from build123d import *

# Parameters (mm, degrees)
SKETCH_15_W          = 13
SKETCH_15_H          = 25
EXTRUDE_4_DEPTH      = 20
CUT_EXTRUDE_START    = 1
SKETCH_16_W          = 12
SKETCH_16_H          = 23
CUT_EXTRUDE_47_DEPTH = 24.6018292
CUT_EXTRUDE_48_DEPTH = 25.6018292


with BuildPart() as part:
    # 스케치15 → 보스-돌출4 (new body)
    with BuildSketch(Plane(origin=(0, 0, 0), x_dir=(1, 0, 0), z_dir=(0, 1, 0))):
        with Locations((0.5, 0)):
            Rectangle(SKETCH_15_W, SKETCH_15_H)
    extrude(amount=EXTRUDE_4_DEPTH)

    # 스케치16 → 컷-돌출47 (cut, through all)
    with BuildSketch(Plane(origin=(0, 0, 0), x_dir=(1, 0, 0), z_dir=(0, 1, 0)).offset(CUT_EXTRUDE_START)):
        with Locations((1, 0)):
            Rectangle(SKETCH_16_W, SKETCH_16_H)
    extrude(amount=CUT_EXTRUDE_47_DEPTH, mode=Mode.SUBTRACT)

    # 스케치17 → 컷-돌출48 (cut, through all)
    with BuildSketch(Plane(origin=(0, 0, 0), x_dir=(1, 0, 0), z_dir=(0, 1, 0))):
        with BuildLine():
            Line((-5, 2.5), (7, 2.5))
            Line((7, 2.5), (7, -5.5))
            ThreePointArc((7, -5.5), (1, -11.5), (-5, -5.5))
            Line((-5, -5.5), (-5, 2.5))
        make_face()
    extrude(amount=CUT_EXTRUDE_48_DEPTH, mode=Mode.SUBTRACT)


solid = part.part
Model file for the job. Use its own axes, mm. A direction names the side the tool comes from. Give positions to 0.01 mm unless a question says otherwise; leave off trailing zeros. Loops run counter-clockwise (first coordinate to the right, second up) from the corner with the lowest first, then second, coordinate; pieces in that order, holes last. Notation, with made-up numbers: (-29, -20.75) -> (-9, -20.75) arc R30 ccw to (-9, 15.25) -> close; hole circle Ø9 at (15.25, 48.5). An arc over 180 degrees is marked (long way). Use a Markdown table: item, result. Add a question column.
(1) Slice it at B-B on z = 10.75. List the corners of the cut face in (x, y).
(2) Slice it at D-D on z = -8. List the corners of the cut face in (x, y).
(3) Drop a flat-ended pin along its axis: pin 1 Ø4.5 at (x, z) = (3.5, -8.5) entering from +Y. Give the stop position or say it passes through.
(4) Slice it at C-C on y = 13.5. List the corners of the cut face in (x, z), and give its area (3 significant figures).
(5) Slice it at A-A on x = -4.25. List the corners of the cut face in (y, z), and give its area (3 significant figures).
(6) Wall check: line 1 along Z through (x, y) = (5.75, 15.25); line 2 along X through (y, z) = (7, 7); line 3 along Y through (x, z) = (-4.75, -7.5). Give the ranges that are in metal, low to high.
(7) Tool access for faces 1 (the flat face through (0.9, 0.5, -2.5)), 2 (the flat face through (0, 10, 12.5)), 3 (the flat face through (6, 1, 10)): list every direction of +Z, -Z, +X, -X, +Y, -Y with a clear straight run to the whole face (end or side of a thin tool).
(8) Mould opens along X. For faces 4 (the cylindrical face through (1.1, 0.5, 11.5)), 5 (the flat face through (7, 8, 12)), 6 (the flat face through (0, 0, -3)) say: +X half, -X half, draft (parallel to the pull), parting line (faces both ways), or undercut.
Filled sheet:
| question | item | result |
|---|---|---|
| 1 | outline | (-6, 0) -> (-1.9, 0) -> (-1.9, 1) -> (-5, 1) -> (-5, 20) -> (-6, 20) -> close; (3.9, 0) -> (7, 0) -> (7, 1) -> (3.9, 1) -> close |
| 2 | outline | (-6, 0) -> (7, 0) -> (7, 1) -> (-5, 1) -> (-5, 20) -> (-6, 20) -> close |
| 3 | pin 1 | y = 1 |
| 4 | outline | (-6, -12.5) -> (7, -12.5) -> (7, -11.5) -> (-5, -11.5) -> (-5, 11.5) -> (7, 11.5) -> (7, 12.5) -> (-6, 12.5) -> close |
| 4 | area | 49.0 mm2 |
| 5 | outline | (0, -12.5) -> (20, -12.5) -> (20, -11.5) -> (1, -11.5) -> (1, -2.5) -> (0, -2.5) -> close; (0, 8.4) -> (1, 8.4) -> (1, 11.5) -> (20, 11.5) -> (20, 12.5) -> (0, 12.5) -> close |
| 5 | area | 52.1 mm2 |
| 6 | line 1 | -12.5 to -11.5, 11.5 to 12.5 |
| 6 | line 2 | -6 to -5 |
| 6 | line 3 | 0 to 1 |
| 7 | face 1 | +X, +Y, -Y |
| 7 | face 2 | +Z, +X, -X, +Y, -Y |
| 7 | face 3 | +X, +Y |
| 8 | face 4 | undercut |
| 8 | face 5 | +X half |
| 8 | face 6 | draft |
